Verification items for this drawing (mm, ordinates from the low corner). A direction names the side the tool comes from. Give positions to 0.01 mm unless a question says otherwise; leave off trailing zeros. Order: outer loops, then holes, each group sorted by start corner. A loop starts at its lowest first (then second) coordinate and runs counter-clockwise, first axis right, second up. Notation, with made-up numbers: M 78,76.25 L 97,76.25 A18 ccw 97,82.25 Z; hole C -15.75,76.5 d2. An arc over 180 degrees is marked long. Answer as a JSON object with one key per item and string values.
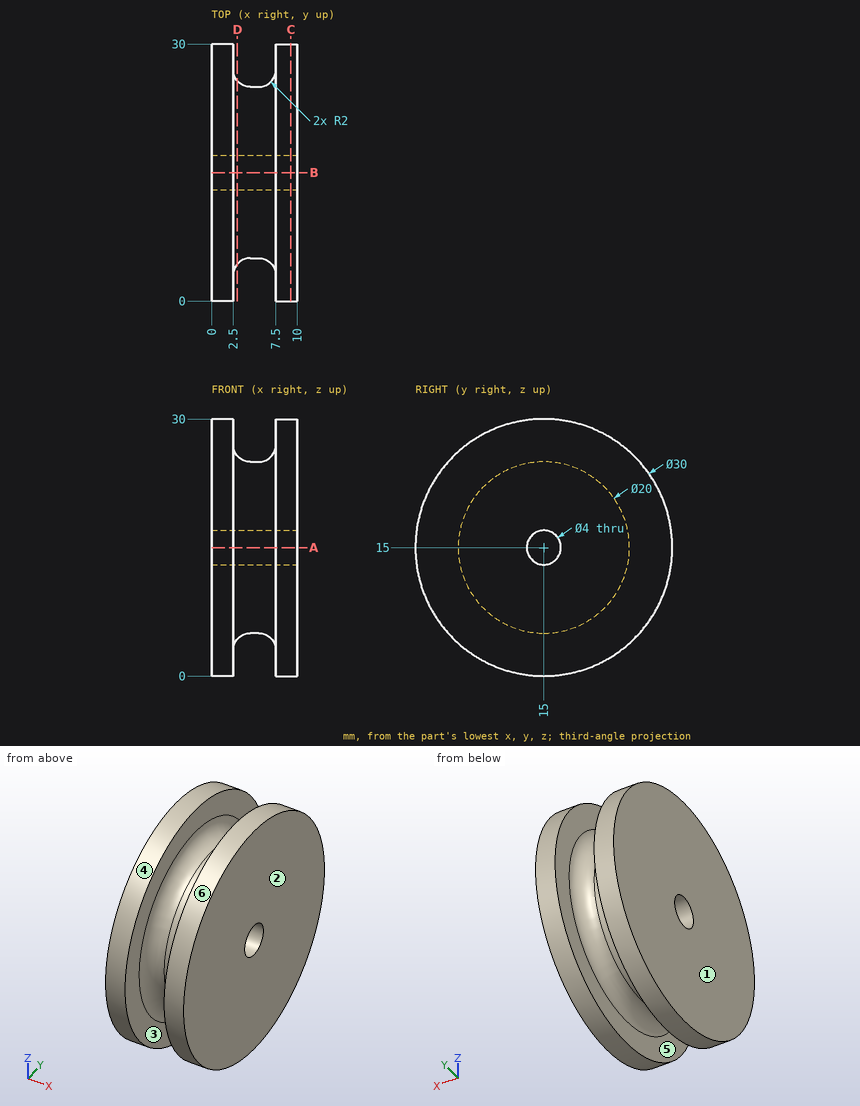
Q1. Gauge pin test, flat ends, axial feed: pin 1 Ø3 at (x, z) = (8.5, 6.5) entering from +Y; pin 2 Ø1.5 at (x, y) = (1.5, 25) entering from -Z. Record the tip position at first contact, or that the pin passes through.
Resolved:
{"pin 1": "stops at y = 28.27", "pin 2": "stops at z = 3.19"}
Q2. Section check D-D on x = 3. Record the cut outline in (y, z).
Resolved:
{"outline": "C 15,15 d21.35; hole C 15,15 d4"}
Q3. Section check C-C on x = 9.25. Record the cut outline in (y, z), then the cut area to 3 significant figures.
Resolved:
{"outline": "C 15,15 d30; hole C 15,15 d4", "area": "694 mm²"}
Q4. Material ranges on L1, parallel to X at y = 9.25, z = 4.5; L2, parallel to Y at x = 5.25, z = 15; L3, parallel to X at y = 11.25, z = 24.5, recorded low to high.
Resolved:
{"L1": "x = 0 to 2.5, 7.5 to 10", "L2": "y = 5 to 13, 17 to 25", "L3": "x = 0 to 3.6, 6.4 to 10"}
Q5. Tool access check on the marked faces 5 and 6. Record the directions out of +Z, -Z, +X, -X, +Y, -Y that give a thin tool (end or side, any length) a straight path to the whole face; none if there is none.
Resolved:
{"face 5": "none", "face 6": "+X, -X"}
Q6. Section check A-A on z = 15. Record the cut outline in (x, y), then the cut area to 3 significant figures.
Resolved:
{"outline": "M 0,0 L 2.5,0 L 2.5,3 A2 cw 4.5,5 L 5.5,5 A2 cw 7.5,3 L 7.5,0 L 10,0 L 10,13 L 0,13 Z; M 0,17 L 10,17 L 10,30 L 7.5,30 L 7.5,27 A2 cw 5.5,25 L 4.5,25 A2 cw 2.5,27 L 2.5,30 L 0,30 Z", "area": "213 mm²"}
Q7. Release check for a two-part mould opening along X. For the marked faces 1, 2, 3 and 4 record: +X half, -X half, draft (parallel to the pull), parting line (faces both ways), or undercut.
Resolved:
{"face 1": "-X half", "face 2": "+X half", "face 3": "undercut", "face 4": "draft"}
